For this review, use the dimensioned drawing (mm, ordinates from the lowest corner) and the shaded views. A direction names the side the tool comes from. Coordinates: 2 decimals unless noted, no trailing zeros. Loops run counter-clockwise (first coordinate to the right, second up) from the corner with the lowest first, then second, coordinate; pieces in that order, holes last. Notation, with made-up numbers: (50, 78.5) - (84, 78.5) arc R20 cw to (84, 106.5) - close; hole circle Ø11 at (-13, 12). An arc over 180 degrees is marked (long way). Return JSON: item names as keys, results as strings. Group by question number.
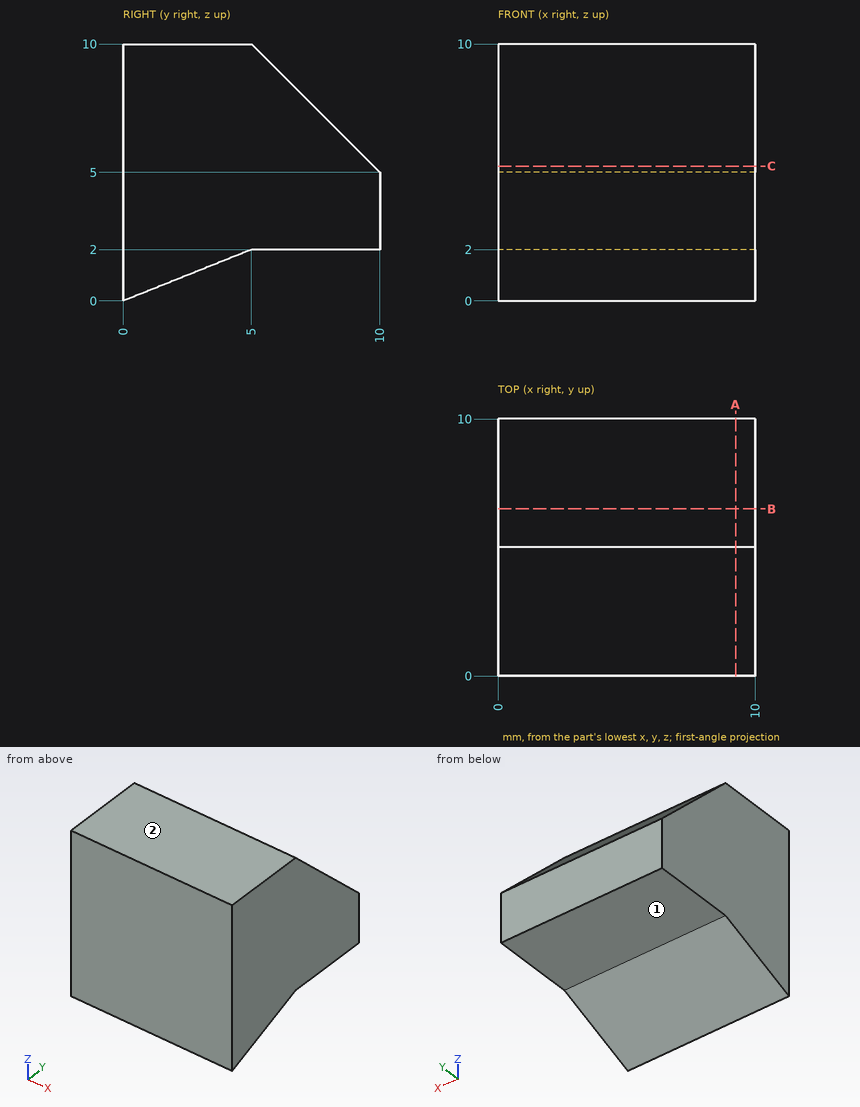
Item 1: Add section C-C (z = 5.25). State the section outline as (x, y) points.
Item 2: To check wall thickness, follow line 1 (Y direction, x = 1.5, z = 9.25); line 2 (Y direction, x = 4, z = 5.5); line 3 (Z direction, x = 9.75, y = 8.5). State the ranges of each line that lie inside material, in increasing order. Write a range as from..to.
Item 3: Add section B-B (y = 6.5). State the section outline as (x, z) points, then the cut area to 3 significant figures.
Item 4: For the marked faces 1 and 2, list the 3-axis set-ups (+Z, -Z, +X, -X, +Y, -Y) from which the entire face can be reached by the end or side of a thin tool; tool diameter is ignored.
Item 5: For P1, Ø4, axis at x = 4.5, y = 8.5, coming from the -Z side, flat-tipped, find the tip position at first contact; note if it passes through.
Item 6: Add section A-A (x = 9.25). State the section outline as (y, z) points.
Answers below:
{
 "1": {"outline": "(0, 0) - (10, 0) - (10, 9.75) - (0, 9.75) - close"},
 "2": {"line 1": "y = 0..5.75", "line 2": "y = 0..9.5", "line 3": "z = 2..6.5"},
 "3": {"outline": "(0, 2) - (10, 2) - (10, 8.5) - (0, 8.5) - close", "area": "65.0 mm^2"},
 "4": {"face 1": "-Z, +X, -X, +Y", "face 2": "+Z, +X, -X, +Y, -Y"},
 "5": {"P1": "stops at z = 2"},
 "6": {"outline": "(0, 0) - (5, 2) - (10, 2) - (10, 5) - (5, 10) - (0, 10) - close"}
}
